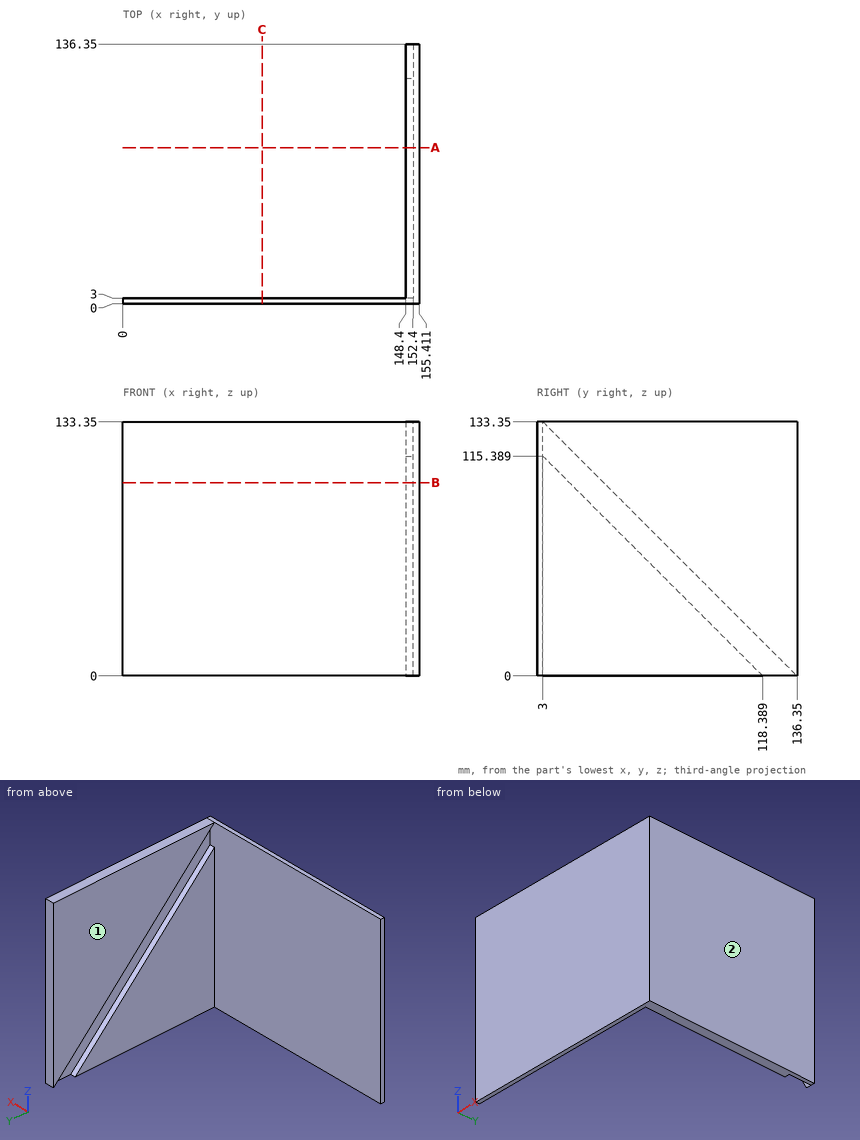
Check sheet for the drawn part. Datum: minimum x, y, z corner. Units: mm. A direction names the side the tool comes from. Round coordinates to 2 decimals unless told otherwise and drop trailing zeros. Loops run counter-clockwise (first coordinate to the right, second up) from the corner with the lowest first, then second, coordinate; pieces in that order, holes last. Notation, with made-up numbers: (50, -8.5) -> (63, -8.5) arc R20 cw to (63, 14.5) -> close; hole circle Ø4 at (89.5, 22.25). An arc over 180 degrees is marked (long way). Put each result on its own line as item: value. Start each with the question number.
1. Gauge pin test, flat ends, axial feed: pin 1 (5 mm diameter, centred on x = 50.5, z = 99.5, fed in from +Y); pin 2 (12 mm diameter, centred on x = 59, z = 23.5, fed in from -Y); pin 3 (3 mm diameter, centred on y = 53, z = 65, fed in from -X). Record the tip position at first contact, or that the pin passes through.
2. Section check A-A (y = 82). Enter the section's corners in (x, z), plus the area to 3 significant figures.
3. Section check C-C (x = 73). Enter the section's corners in (y, z).
4. Access from +Z, -Z, +X, -X, +Y, -Y to the whole of each face (thin tool, end or side, straight path). Record for the marked faces 1 and 2.
5. Scan lines: probe 1 along Y at (x, z) = (114, 44.5); probe 2 along X at (y, z) = (52, 79.5); probe 3 along X at (y, z) = (54, 85). Record each from-to range of solid material in increasing order.
6. Section check B-B (z = 101.5). Enter the section's corners in (x, y).
Findings:
1. pin 1: stops at y = 3
1. pin 2: stops at y = 0
1. pin 3: stops at x = 148.4
2. outline: (148.4, 0) -> (155.41, 0) -> (155.41, 133.35) -> (148.4, 133.35) -> (148.4, 54.35) -> (152.4, 54.35) -> (152.4, 36.39) -> (148.4, 36.39) -> close
2. area: 863 mm^2
3. outline: (0, 0) -> (3, 0) -> (3, 133.35) -> (0, 133.35) -> close
4. face 1: +Z, -Z, -X, +Y
4. face 2: +Z, -Z, +X, +Y, -Y
5. probe 1: y = 0 to 3
5. probe 2: x = 152.4 to 155.41
5. probe 3: x = 148.4 to 155.41
6. outline: (0, 0) -> (155.41, 0) -> (155.41, 136.35) -> (148.4, 136.35) -> (148.4, 34.85) -> (152.4, 34.85) -> (152.4, 16.89) -> (148.4, 16.89) -> (148.4, 3) -> (0, 3) -> close
